Model file for the job. Use its own axes, mm. Coordinates: 2 decimals unless noted, no trailing zeros. Write each loop counter-clockwise with the first axis right and the second up, starting at its lowest first coordinate (ties: lowest second). Pieces come first, ordered by that corner, then holes. Notation, with made-up numbers: M 64,34 L 70,34 A3 cw 70,38 Z; hole C 41.25,-6 d3. An arc over 180 degrees is marked long. Put each result on its own line as item: value. Start each with the question number.
Q1. Cut at D-D (y = -4.5). Write the cut outline in (x, z), then the cut area to 3 significant figures.
Q2. Drop flat-ended pins along their axis: pin 1 (1 mm diameter, centred on x = 55.5, y = 0.5, fed in from -Z); pin 2 (5 mm diameter, centred on x = 26, z = 1.5, fed in from -Y); pin 3 (3 mm diameter, centred on x = 91, y = -2, fed in from +Z); pin 4 (5.5 mm diameter, centred on y = -2.5, z = 1, fed in from -X). Give the stop position or say it passes through.
Q3. Cut at C-C (x = 22.5). Write the cut outline in (y, z).
Q4. Cut at A-A (y = 0). Write the cut outline in (x, z).
Q5. Drill centre lines: line 1 along Y through (x, z) = (13.5, -0.25); line 2 along Y through (x, z) = (91, -1); line 3 along X through (y, z) = (1.25, 3). Where is each one in solid material? Low to high.
Autodesk Inventor part; units mm, degrees
ref_plane "dia1_XY" through (0, 2.3749, 0) normal (1, 0, 0) x (0, 0, -1)
ref_plane "dia1_YZ" through (0, 2.3749, 0) normal (0, 0, -1) x (0, 1, 0)
ref_plane "dia1_ZX" through (0, 2.3749, 0) normal (0, 1, 0) x (1, 0, 0)
sketch "Sketch_1" plane through (0, 0, 0) normal (0, 0, 1) x (1, 0, 0)
  line L0 (104.6988, 0) -> (0, 0)
  line L1 (0, 0) -> (0, 2.3749)
  line L2 (0, 2.3749) -> (93.6752, 2.3749)
  line L3 (93.6752, 2.3749) -> (93.6752, 5.6197)
  line L4 (93.6752, 5.6197) -> (104.6988, 5.6197)
  line L5 (104.6988, 5.6197) -> (104.6988, 0)
  line L6 (104.6988, 0) -> (0, 0)
revolve "Revolution1" add sketch "Sketch_1" angle 360 about axis through (104.6988, 0, 0) along (1, 0, 0)
sketch "Sketch_3" plane through (0, 0, 0) normal (0, 0, 1) x (1, 0, 0)
  line L0 (0, 0) -> (-12.7, 0)
  line L1 (-12.7, 0) -> (-12.7, 1.9406)
  line L2 (-12.7, 1.9406) -> (-12.2276, 2.413)
  line L3 (-12.2276, 2.413) -> (0, 2.413)
  line L4 (0, 2.413) -> (0, 0)
  line L5 (0, 0) -> (-12.7, 0)
revolve "Revolution2" add sketch "Sketch_3" angle 360 about axis through (0, 0, 0) along (1, 0, 0)
thread "Thread1"
sketch "Sketch_30" plane through (0, 0, 0) normal (0, 0, 1) x (1, 0, 0)
  line L0 (0, 0) -> (-0.254, 0)
  line L1 (-0.254, 2.667) -> (-0.254, 2.159)
  line L2 (-0.254, 2.159) -> (0, 2.159)
  line L3 (0, 2.159) -> (0, 2.667)
  line L4 (0, 2.667) -> (-0.254, 2.667)
revolve "Revolution3" cut sketch "Sketch_30" angle 360 about axis through (0, 0, 0) along (1, 0, 0)
ref_plane "dia1_XY" through (0, 2.3749, 0) normal (1, 0, 0) x (0, 0, -1)
ref_plane "dia1_YZ" through (0, 2.3749, 0) normal (0, 0, -1) x (0, 1, 0)
ref_plane "dia1_ZX" through (0, 2.3749, 0) normal (0, 1, 0) x (1, 0, 0)
ref_plane "dia12_XY" through (0, 0, 9.3726) normal (1, 0, 0) x (0, 0, -1)
ref_plane "dia12_YZ" through (0, 0, 9.3726) normal (0, 0, -1) x (0, 1, 0)
ref_plane "dia12_ZX" through (0, 0, 9.3726) normal (0, 1, 0) x (1, 0, 0)
ref_plane "dia2_XY" through (0, -2.3749, 0) normal (1, 0, 0) x (0, 0, -1)
ref_plane "dia2_YZ" through (0, -2.3749, 0) normal (0, 0, -1) x (0, 1, 0)
ref_plane "dia2_ZX" through (0, -2.3749, 0) normal (0, 1, 0) x (1, 0, 0)
ref_plane "dia22_XY" through (0, 0, -9.3726) normal (1, 0, 0) x (0, 0, -1)
ref_plane "dia22_YZ" through (0, 0, -9.3726) normal (0, 0, -1) x (0, 1, 0)
ref_plane "dia22_ZX" through (0, 0, -9.3726) normal (0, 1, 0) x (1, 0, 0)
ref_plane "rl1_XY" through (-12.7, 0, 0) normal (1, 0, 0) x (0, 0, -1)
ref_plane "rl1_YZ" through (-12.7, 0, 0) normal (0, 0, -1) x (0, 1, 0)
ref_plane "rl1_ZX" through (-12.7, 0, 0) normal (0, 1, 0) x (1, 0, 0)
ref_plane "rl2_XY" through (0, 0, 0) normal (1, 0, 0) x (0, 0, -1)
ref_plane "rl2_YZ" through (0, 0, 0) normal (0, 0, -1) x (0, 1, 0)
ref_plane "rl2_ZX" through (0, 0, 0) normal (0, 1, 0) x (1, 0, 0)
ref_plane "rod_cp_XY" through (0, 0, 0) normal (1, 0, 0) x (0, 0, -1)
ref_plane "rod_cp_YZ" through (0, 0, 0) normal (0, 0, -1) x (0, 1, 0)
ref_plane "rod_cp_ZX" through (0, 0, 0) normal (0, 1, 0) x (1, 0, 0)
ref_plane "thd1_XY" through (-12.7, 2.413, 0) normal (1, 0, 0) x (0, 0, -1)
ref_plane "thd1_YZ" through (-12.7, 2.413, 0) normal (0, 0, -1) x (0, 1, 0)
ref_plane "thd1_ZX" through (-12.7, 2.413, 0) normal (0, 1, 0) x (1, 0, 0)
ref_plane "thd2_XY" through (-12.7, -2.413, 0) normal (1, 0, 0) x (0, 0, -1)
ref_plane "thd2_YZ" through (-12.7, -2.413, 0) normal (0, 0, -1) x (0, 1, 0)
ref_plane "thd2_ZX" through (-12.7, -2.413, 0) normal (0, 1, 0) x (1, 0, 0)
ref_plane "to_rod_clevis_XY" through (-12.7, 0, 0) normal (1, 0, 0) x (0, 0, -1)
ref_plane "to_rod_clevis_YZ" through (-12.7, 0, 0) normal (0, 0, -1) x (0, 1, 0)
ref_plane "to_rod_clevis_ZX" through (-12.7, 0, 0) normal (0, 1, 0) x (1, 0, 0)
properties part number "012.5-DP0_rod"
Computed values:
1. outline: M 93.68,-3.37 L 104.7,-3.37 L 104.7,3.37 L 93.68,3.37 Z
1. area: 74.2 mm2
2. pin 1: z = -2.37
2. pin 2: y = -2.37
2. pin 3: z = 2.32
2. pin 4: x = -12.7
3. outline: C 0,0 d4.75
4. outline: M -12.7,-1.94 L -12.23,-2.41 L -0.25,-2.41 L -0.25,-2.16 L 0,-2.16 L 0,-2.37 L 93.68,-2.37 L 93.68,-5.62 L 104.7,-5.62 L 104.7,5.62 L 93.68,5.62 L 93.68,2.37 L 0,2.37 L 0,2.16 L -0.25,2.16 L -0.25,2.41 L -12.23,2.41 L -12.7,1.94 Z
5. line 1: -2.36 to 2.36
5. line 2: -2.15 to 2.15
5. line 3: 93.68 to 104.7
